For this review, use the dimensioned drawing (mm, ordinates from the lowest corner) and the shaded views. A direction names the side the tool comes from. Round coordinates to 2 decimals unless told otherwise and drop trailing zeros. Order: outer loops, then holes, each group sorted by start corner. A loop starts at its lowest first (then second) coordinate and runs counter-clockwise, first axis right, second up. Notation, with made-up numbers: (85, -30.75) - (89, -30.75) arc R21 cw to (89, 1.25) - close; hole circle Ø1 at (3, -40). An arc over 180 degrees is marked (long way). Use CSV: the item, a comma, the result in double quotes. Start each with the question number.
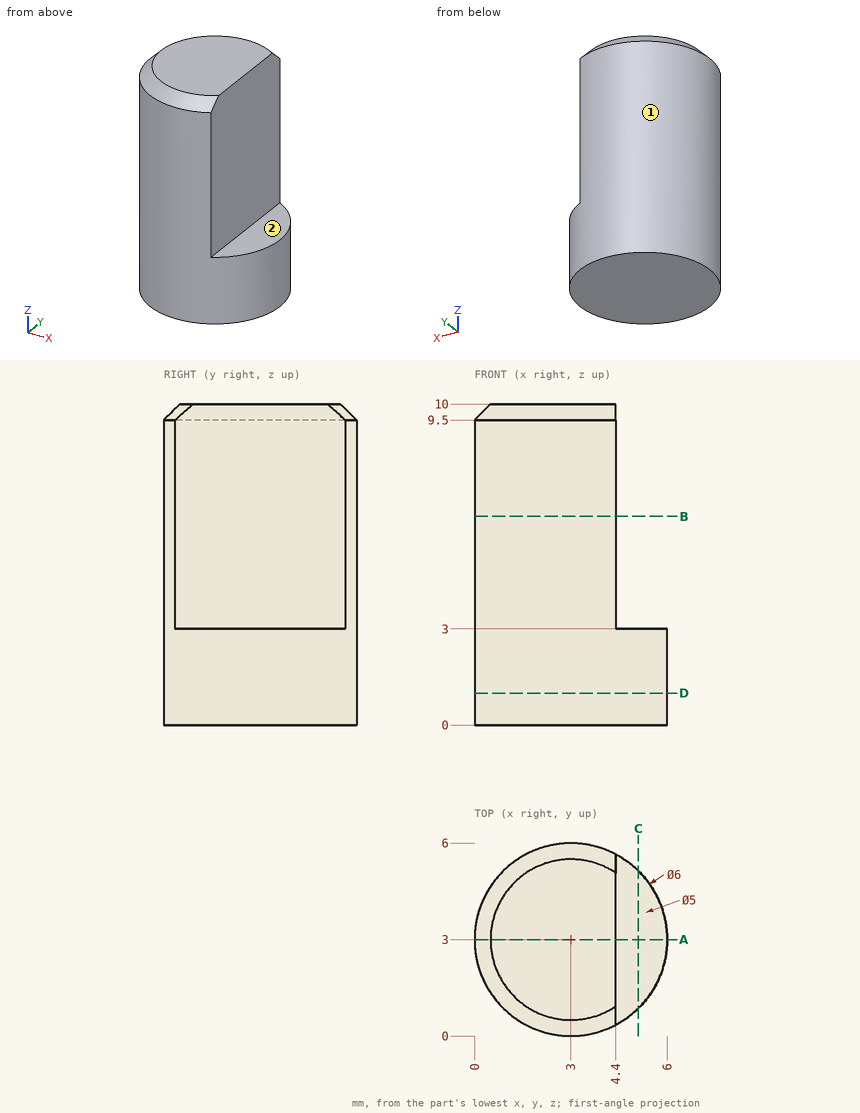
Q1. Take a section at B-B (z = 6.5). State the section outline as (x, y) points, plus the area to 3 significant figures.
Q2. Take a section at C-C (x = 5.1). State the section outline as (y, z) points.
Q3. Clearance check with flat-ended pins moving along their axes: pin 1 (1.5 mm diameter, centred on x = 5, z = 7, fed in from +Y); pin 2 (0.5 mm diameter, centred on x = 5.5, y = 2.5, fed in from +Z); pin 3 (2.5 mm diameter, centred on y = 2, z = 7, fed in from +X). State where each tip first meets the part, or that it passes through.
Q4. Take a section at D-D (z = 1). State the section outline as (x, y) points.
Q5. For L1, parallel to X at y = 2.9, z = 9; L2, parallel to Z at x = 5.05, y = 2.3; L3, parallel to Y at x = 2.15, z = 7, list the stretches that pass through material, from the lowest coordinate up. Write a range as [from, to].
Q6. Take a section at A-A (y = 3). State the section outline as (x, z) points.
Q7. Tool access review of the marked faces 1 and 2: name each direction out of +Z, -Z, +X, -X, +Y, -Y from which nothing blocks a thin tool from reaching the whole face with its end or side.
Findings below:
1,outline,"(4.4, 0.35) - (4.4, 5.65) arc R3 ccw (long way) to start"
1,area,"22.2 mm^2"
2,outline,"(0.86, 0) - (5.14, 0) - (5.14, 3) - (0.86, 3) - close"
3,pin 1,"stops at y = 5.73"
3,pin 2,"stops at z = 3"
3,pin 3,"stops at x = 4.4"
4,outline,"circle Ø6 at (3, 3)"
5,L1,"x = [0, 4.4]"
5,L2,"z = [0, 3]"
5,L3,"y = [0.12, 5.88]"
6,outline,"(0, 0) - (6, 0) - (6, 3) - (4.4, 3) - (4.4, 10) - (0.5, 10) - (0, 9.5) - close"
7,face 1,"+Z, -Z"
7,face 2,"+Z, +X, +Y, -Y"
